The model under review builds one solid part; all positions refer to its coordinate system, in mm. Face numbers are marked on the shaded views. Coordinates: 2 decimals unless noted, no trailing zeros. Order: outer loops, then holes, each group sorted by start corner. A loop starts at its lowest first (then second) coordinate and runs counter-clockwise, first axis right, second up.
```python
from build123d import *

# Parameters (mm, degrees)
SKETCH1_W                   = 22.225
SKETCH1_H                   = 57.15
BOSS_EXTRUDE1_DEPTH         = 12.7
F_1_4_0_25_DIAMETER_HOLE1_D = 6.35


with BuildPart() as part:
    # Sketch1 → Boss-Extrude1 (new body)
    with BuildSketch(Plane.XY):
        with Locations((-11.1125, 28.575)):
            Rectangle(SKETCH1_W, SKETCH1_H)
    extrude(amount=-BOSS_EXTRUDE1_DEPTH)

    # 1/4 (0.25) Diameter Hole1 (through all)
    with Locations(Plane.XY):
        with Locations((-17.4625, 47.625), (-17.4625, 28.575), (-17.4625, 9.525)):
            Hole(F_1_4_0_25_DIAMETER_HOLE1_D / 2)


solid = part.part
```
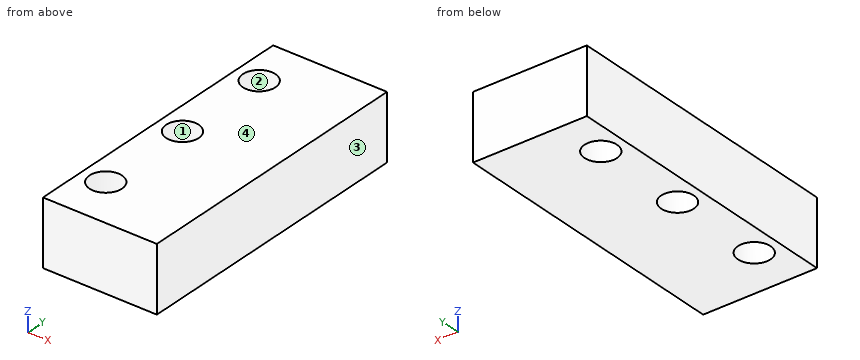
(1) We need section A-A, the plane x = -17. Write out the cut boundary in (y, z), and give its area (3 significant figures).
A:
outline: (0, -12.7) - (6.38, -12.7) - (6.38, 0) - (0, 0) - close; (12.67, -12.7) - (25.43, -12.7) - (25.43, 0) - (12.67, 0) - close; (31.72, -12.7) - (44.48, -12.7) - (44.48, 0) - (31.72, 0) - close; (50.77, -12.7) - (57.15, -12.7) - (57.15, 0) - (50.77, 0) - close
area: 486 mm2
(2) Wall thickness on probe 1 along X at (y, z) = (28, -10.25) (3 decimals); probe 2 along Y at (x, z) = (-15, -12); probe 3 along Y at (x, z) = (-16.25, -9.25): over which ranges is each line inside the solid? List them lowest first.
A:
probe 1: x = -22.225 to -20.585, -14.34 to 0
probe 2: y = 0 to 7.52, 11.53 to 26.57, 30.58 to 45.62, 49.63 to 57.15
probe 3: y = 0 to 6.59, 12.46 to 25.64, 31.51 to 44.69, 50.56 to 57.15
(3) For pin 1 Ø3 at (x, z) = (-5.5, -8.5) entering from -Y, flat-tipped, find the tip position at first contact; note if it passes through.
A:
pin 1: stops at y = 0
(4) We need section B-B, the plane y = 7. Write out the cut boundary in (x, z) (3 decimals).
A:
outline: (-22.225, -12.7) - (-19.387, -12.7) - (-19.387, 0) - (-22.225, 0) - close; (-15.538, -12.7) - (0, -12.7) - (0, 0) - (-15.538, 0) - close
(5) We need section C-C, the plane z = -11.25. Count the separate pieces of the cut face and the enclosed holes in it, and give its area (3 significant figures).
A:
separate pieces: 1
enclosed holes: 3
area: 1,180 mm2
(6) Draft analysis for pull direction X (two halves, no side actions). For the marked faces 1, 2, 3 and 4, state which applies: released by +X, released by -X, zero draft, split by the parting line, or undercut.
A:
face 1: undercut
face 2: undercut
face 3: released by +X
face 4: zero draft
